```python
from build123d import *

# Parameters (mm, degrees)
F0_R     = 25.4
F1_DEPTH = 1069.975
F2_W     = 50.8
F2_H     = 152.4
F3_DEPTH = 3.175
F5_D     = 15.875
F7_DEPTH = 3.175
F9_D     = 15.875


with BuildPart() as f1:
    # F0 (on Right) → F1 (new body)
    with BuildSketch(Plane.YZ):
        Circle(F0_R)
    extrude(amount=F1_DEPTH)

    # F2 (on Right) → F3 (join)
    with BuildSketch(Plane.YZ):
        Rectangle(F2_W, F2_H)
    extrude(amount=F3_DEPTH)

    # F5 (through all)
    with Locations(Plane(origin=(0, 0, 0), x_dir=(0, -1, 0), z_dir=(-1, 0, 0))):
        with Locations((0, 50.8), (0, -50.8)):
            Hole(F5_D / 2)

    # F6 (on face) → F7 (join)
    with BuildSketch(Plane.YZ.offset(1069.975)):
        Polygon((25.4, 0), (25.4, 76.2), (-25.4, 76.2), (-25.4, 0), (-25.4, -76.2), (25.4, -76.2), align=None)
    extrude(amount=-F7_DEPTH)

    # F9 (through all)
    with Locations(Plane.YZ.offset(1069.975)):
        with Locations((0, 50.8), (0, -50.8)):
            Hole(F9_D / 2)


solid = f1.part
```
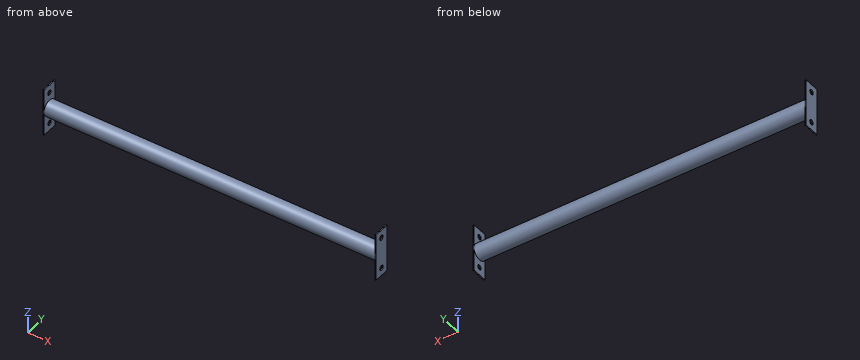
Can you work these out from the model? Positions are in its coordinate system, mm. Coordinates: 2 decimals unless noted, no trailing zeros. Order: outer loops, then holes, each group sorted by start corner. A loop starts at its lowest first (then second) coordinate and runs counter-clockwise, first axis right, second up. Notation, with made-up numbers: (87.5, 16) -> (119.5, 16) arc R24 cw to (119.5, 30) -> close; hole circle Ø6 at (53.5, 32.5). An arc over 180 degrees is marked (long way). Write each question's results on one line, items separated by ' | '.
Item 1: If I drill on line 1 along Z through (x, y) = (2.5, 0); line 2 along X through (y, z) = (22.5, 47) (3 decimals); line 3 along Y through (x, z) = (0.8, -50.8), over which ranges is the centre line in solid material (lowest first)?
Results are:
line 1: -76.2 to -58.74, -42.86 to 42.86, 58.74 to 76.2 | line 2: 0 to 3.175, 1066.8 to 1069.975 | line 3: -25.4 to -7.94, 7.94 to 25.4
Item 2: I'm going to push flat-ended pins straight in: pin 1 Ø15 at (y, z) = (1.5, -53.5) entering from -X; pin 2 Ø3 at (x, z) = (610, -11.5) entering from +Y; pin 3 Ø1.5 at (x, y) = (146, -17) entering from -Z; pin 4 Ø5 at (x, z) = (553, 17) entering from +Y. Where does each tip first touch, or does it pass through?
Results are:
pin 1: x = 0 | pin 2: y = 23.35 | pin 3: z = -19.52 | pin 4: y = 20.85
Item 3: I want a section at A-A, the plane y = 0. Write out the boundary of the cut face in (x, z) (1 decimal), then the cut area to 3 significant figures.
Results are:
outline: (0, -76.2) -> (3.2, -76.2) -> (3.2, -58.7) -> (0, -58.7) -> close; (0, -42.9) -> (3.2, -42.9) -> (3.2, -25.4) -> (1066.8, -25.4) -> (1066.8, -42.9) -> (1070, -42.9) -> (1070, 42.9) -> (1066.8, 42.9) -> (1066.8, 25.4) -> (3.2, 25.4) -> (3.2, 42.9) -> (0, 42.9) -> close; (0, 58.7) -> (3.2, 58.7) -> (3.2, 76.2) -> (0, 76.2) -> close; (1066.8, -76.2) -> (1070, -76.2) -> (1070, -58.7) -> (1066.8, -58.7) -> close; (1066.8, 58.7) -> (1070, 58.7) -> (1070, 76.2) -> (1066.8, 76.2) -> close | area: 54,800 mm²
Item 4: I want a section at B-B, the plane x = 904. Write out the boundary of the cut face in (y, z), then the cut area to 3 significant figures.
Results are:
outline: circle Ø50.8 at (0, 0) | area: 2,030 mm²
